The model under review builds one solid part; all positions refer to its coordinate system, in mm. A direction names the side the tool comes from. Round coordinates to 2 decimals unless told otherwise and drop trailing zeros. Order: outer loops, then holes, each group sorted by start corner. A loop starts at its lowest first (then second) coordinate and runs counter-clockwise, first axis right, second up.
from build123d import *

# Parameters (mm, degrees)
SKETCH_1_W           = 27
SKETCH_1_H           = 16.5
EXTRUDE_1_DEPTH      = 4
SKETCH_2_R           = 1.1
CUT_EXTRUDE_1_DEPTH  = 4
SKETCH_3_R           = 4.8
EXTRUDE_2_DEPTH      = 10
EXTRUDE_3_DEPTH      = 13
FILLET_1_R           = 0.5
FILLET_2_R           = 1
EXTRUDE_4_REACH      = 29.807
EXTRUDE_4_END_RADIUS = 4.8
SKETCH_7_R           = 1.3
CUT_EXTRUDE_3_DEPTH  = 7
CHAMFER_1_SIZE       = 0.4
CHAMFER_1_SIZE2      = 0.692820323
FILLET_3_R           = 0.5
EXTRUDE_5_DEPTH      = 14
FILLET_4_R           = 0.5
CHAMFER_2_SIZE       = 1


with BuildPart() as part:
    # Sketch 1 → Extrude 1 (new body)
    with BuildSketch(Plane.XY):
        with Locations((3.5, 0)):
            Rectangle(SKETCH_1_W, SKETCH_1_H)
    extrude(amount=EXTRUDE_1_DEPTH)

    # Sketch 2 → Cut-Extrude 1 (cut)
    with BuildSketch(Plane.XY.offset(4)):
        with Locations((-8, 0)):
            Circle(SKETCH_2_R)
        Circle(SKETCH_2_R)
    extrude(amount=-CUT_EXTRUDE_1_DEPTH, mode=Mode.SUBTRACT)



with BuildPart() as body_2:
    # Sketch 3 → Extrude 2 (new body)
    with BuildSketch(Plane.XZ.offset(8.25)):
        with Locations(Location((9.5, 12, 0), (0, 0, 270))):
            Circle(SKETCH_3_R)
    extrude(amount=-EXTRUDE_2_DEPTH)


with BuildPart() as part_1:
    add(part.part)

    add(body_2.part)  # Extrude 3 merges body 2
    # Sketch 4 → Extrude 3 (add)
    with BuildSketch(Plane.XZ.offset(8.25)):
        with BuildLine():
            Line((6.5, 4), (12.5, 4))
            Line((12.5, 4), (12.38, 8.16))
            ThreePointArc((12.38, 8.16), (9.5, 7.2), (6.62, 8.16))
            Line((6.62, 8.16), (6.5, 4))
        make_face()
    extrude(amount=-EXTRUDE_3_DEPTH)

    # Fillet 1
    fillet_1_edges = [part_1.edges().sort_by_distance(p)[0] for p in [
        (6.62, 3.25, 8.16),
        (12.38, 3.25, 8.16),
    ]]
    fillet(fillet_1_edges, radius=FILLET_1_R)

    # Fillet 2
    # the kernel refuses this fillet: 1 mm, written as the material it adds along each edge
    with BuildSketch(Plane(origin=(7.094742907, 1.75, 7.277210748), x_dir=(0.45382209295910925, 0, 0.891092311683932), z_dir=(0.891092311683932, 0, -0.45382209295910925))) as fillet_2_piece_1_section:
        with BuildLine():
            CenterArc((0.5 + FILLET_2_R, -FILLET_2_R), FILLET_2_R, 90, 90)
            Line((0.5, -FILLET_2_R), (0.5, 0))
            Line((0.5, 0), (0.5 + FILLET_2_R, 0))
        make_face()
    fillet_2_piece_1 = revolve(axis=Axis((7.094742907, 1.75, 7.277210748), (0, -1, 0)), revolution_arc=359.64, mode=Mode.PRIVATE)
    fillet_2_piece_1 = split(fillet_2_piece_1, bisect_by=Plane(origin=(6.594950803, 1.75, 7.291627828), z_dir=(0.9995842091710025, 0, -0.02883415987993323)), keep=Keep.TOP, mode=Mode.PRIVATE)
    add(fillet_2_piece_1)
    with BuildSketch(Plane(origin=(7.094742907, 1.75, 7.277210748), x_dir=(0.45382209295910925, 0, 0.891092311683932), z_dir=(0.891092311683932, 0, -0.45382209295910925))) as fillet_2_piece_2_section:
        with BuildLine():
            CenterArc((0.5 + FILLET_2_R, -FILLET_2_R), FILLET_2_R, 90, 90)
            Line((0.5, -FILLET_2_R), (0.5, 0))
            Line((0.5, 0), (0.5 + FILLET_2_R, 0))
        make_face()
    fillet_2_piece_2 = revolve(axis=Axis((7.094742907, 1.75, 7.277210748), (0, -1, 0)), revolution_arc=359.64, mode=Mode.PRIVATE)
    fillet_2_piece_2 = fillet_2_piece_2 & Plane(origin=(9.5, 1.75, 12), x_dir=(0.6, 0, -0.8000000000000002), z_dir=(0, -1, 0)) * Cylinder(4.8, 6, mode=Mode.PRIVATE)
    add(fillet_2_piece_2)
    with BuildSketch(Plane(origin=(11.905257093, 1.75, 7.277210748), x_dir=(-0.45941199618044226, 0, 0.8882232927397824), z_dir=(0.8882232927397824, 0, 0.45941199618044226))) as fillet_2_piece_3_section:
        with BuildLine():
            CenterArc((0.5 + FILLET_2_R, -FILLET_2_R), FILLET_2_R, 90, 90)
            Line((0.5 + FILLET_2_R, 0), (0.5, 0))
            Line((0.5, 0), (0.5, -FILLET_2_R))
        make_face()
    fillet_2_piece_3 = revolve(axis=Axis((11.905257093, 1.75, 7.277210748), (0, -1, 0)), revolution_arc=359.64, mode=Mode.PRIVATE)
    fillet_2_piece_3 = split(fillet_2_piece_3, bisect_by=Plane(origin=(12.405049197, 1.75, 7.291627828), z_dir=(-0.9995842091710025, 0, -0.02883415987993387)), keep=Keep.TOP, mode=Mode.PRIVATE)
    add(fillet_2_piece_3)
    with BuildSketch(Plane(origin=(11.905257093, 1.75, 7.277210748), x_dir=(-0.45941199618044226, 0, 0.8882232927397824), z_dir=(0.8882232927397824, 0, 0.45941199618044226))) as fillet_2_piece_4_section:
        with BuildLine():
            CenterArc((0.5 + FILLET_2_R, -FILLET_2_R), FILLET_2_R, 90, 90)
            Line((0.5 + FILLET_2_R, 0), (0.5, 0))
            Line((0.5, 0), (0.5, -FILLET_2_R))
        make_face()
    fillet_2_piece_4 = revolve(axis=Axis((11.905257093, 1.75, 7.277210748), (0, -1, 0)), revolution_arc=359.64, mode=Mode.PRIVATE)
    fillet_2_piece_4 = fillet_2_piece_4 & Plane(origin=(9.5, 1.75, 12), x_dir=(0.6, 0, -0.8000000000000002), z_dir=(0, -1, 0)) * Cylinder(4.8, 7, mode=Mode.PRIVATE)
    add(fillet_2_piece_4)
    with BuildSketch(Plane(origin=(9.5, 1.75, 12), x_dir=(-0.4538220929591119, 0, -0.8910923116839305), z_dir=(-0.8910923116839305, 0, 0.4538220929591119))) as fillet_2_piece_5:
        with BuildLine():
            CenterArc((4.8 - FILLET_2_R, -FILLET_2_R), FILLET_2_R, 0, 90)
            Line((4.8, -FILLET_2_R), (4.8, 0))
            Line((4.8, 0), (4.8 - FILLET_2_R, 0))
        make_face()
    revolve(axis=Axis((9.5, 1.75, 12), (0, -1, 0)), revolution_arc=53.978342396)

    # Extrude 4: up to this cylinder (the profile starts outside it)
    extrude_4_end = Plane(origin=(9.5, -4.045075, 12), z_dir=(0, -1, 0)) * Cylinder(EXTRUDE_4_END_RADIUS, 70.214, mode=Mode.PRIVATE)
    # Sketch 5 → Extrude 4 (add, up to the surface)
    with BuildSketch(Plane.XY.offset(20.4), mode=Mode.PRIVATE) as extrude_4_sk1:
        with BuildLine():
            Line((6.5, -8.25), (6.5, -2.25))
            ThreePointArc((6.5, -2.25), (9.5, 0.75), (12.5, -2.25))
            Line((12.5, -2.25), (12.5, -8.25))
            Line((12.5, -8.25), (6.5, -8.25))
        make_face()
    extrude_4_tool1 = extrude(extrude_4_sk1.sketch, amount=-EXTRUDE_4_REACH, mode=Mode.PRIVATE) - extrude_4_end
    add(extrude_4_tool1.solids().sort_by_distance((9.5, -4.045075, 20.4))[0])

    # Sketch 7 → Cut-Extrude 3 (cut)
    with BuildSketch(Plane.XY.offset(20.4)):
        with Locations((9.5, -2.25)):
            Circle(SKETCH_7_R)
    extrude(amount=-CUT_EXTRUDE_3_DEPTH, mode=Mode.SUBTRACT)

    # Chamfer 1
    chamfer_1_edges = [part_1.edges().sort_by_distance(p)[0] for p in [
        (8.2, -2.25, 20.4),
    ]]
    chamfer_1_side = [part_1.faces().sort_by_distance(p)[0] for p in [
        (9.5, -4.257679358, 20.4),
    ]]
    chamfer(chamfer_1_edges, length=CHAMFER_1_SIZE, length2=CHAMFER_1_SIZE2, reference=chamfer_1_side[0])

    # Fillet 3
    fillet_3_edges = [part_1.edges().sort_by_distance(p)[0] for p in [
        (6.5, -1.75, 4),
        (12.5, -1.75, 4),
    ]]
    fillet(fillet_3_edges, radius=FILLET_3_R)

    # Sketch 8 → Extrude 5 (add)
    with BuildSketch(Plane(origin=(17, 0, 0), x_dir=(0, 0, -1), z_dir=(1, 0, 0))):
        with BuildLine():
            Line((6.5, 1.75), (17.350889359, 1.75))
            ThreePointArc((17.350889359, 1.75), (18.144565149, 1.050392929), (17.550087952, 0.17519685))
            ThreePointArc((17.550087952, 0.17519685), (8.361036446, -3.17500409), (0, -8.25))
            Line((0, -8.25), (0, 8.25))
            Line((0, 8.25), (6.5, 1.75))
        make_face()
    extrude(amount=-EXTRUDE_5_DEPTH)

    # Fillet 4
    # the kernel refuses this fillet: 0.5 mm, written as the material it adds along each edge
    with BuildSketch(Plane(origin=(3, -8.25, 0), x_dir=(-1, 0, 0), z_dir=(0, 1, 0))) as fillet_4_piece_1_section:
        with BuildLine():
            CenterArc((FILLET_4_R, -FILLET_4_R), FILLET_4_R, 90, 90)
            Line((0, -FILLET_4_R), (0, 0))
            Line((0, 0), (FILLET_4_R, 0))
        make_face()
    fillet_4_piece_1 = extrude(amount=16.5, mode=Mode.PRIVATE)
    fillet_4_piece_1 = fillet_4_piece_1 - Plane(origin=(3, -48.25, -30), x_dir=(0, 0.9685039370078732, 0.24899824095814338), z_dir=(1, 0, 0)) * Cylinder(50, 35, mode=Mode.PRIVATE)
    fillet_4_piece_1 = split(fillet_4_piece_1, bisect_by=Plane(origin=(3, 0, -8.25), z_dir=(0, -0.7071067811865462, 0.7071067811865488)), keep=Keep.TOP, mode=Mode.PRIVATE)
    add(fillet_4_piece_1)

    # Chamfer 2
    chamfer_2_edges = [part_1.edges().sort_by_distance(p)[0] for p in [
        (-10, 8.25, 2),
        (17, 8.25, 2),
        (17, -8.25, 2),
        (-10, -8.25, 2),
    ]]
    chamfer(chamfer_2_edges, length=CHAMFER_2_SIZE)


solid = part_1.part
(1) To check wall thickness, follow L1, parallel to Y at x = 9.5, z = 17.25; L2, parallel to Y at x = -8, z = 1.85; L3, parallel to X at y = 1.5, z = -1.5. State the ranges of each line that lie inside material, in increasing order.
(2) Clearance check with flat-ended pins moving along their axes: P1, Ø3, axis at x = -5, y = 2, coming from the -Z side; P2, Ø5, axis at x = 1.5, y = -0.5, coming from the +Z side; P3, Ø4, axis at y = 4.5, z = 6.5, coming from the +X side; P4, Ø1.3, axis at x = 0, y = 0, coming from the +Z side. State where each tip first meets the part, or that it passes through.
(3) The part is to be moulded in two halves that separate along Z. For faces 1 (the flat face through (-4, 0, 0)), 2 (the cylindrical face through (5.6, -3.3, 9.2)), 3 (the flat face through (12.5, -5, 18)), 4 (the flat face through (10, -5, 20.4)), say which applies: pulls with the +Z half, pulls with the -Z half, needs draft (parallel to the pull), parting line crosses it, or undercut.
(4) We need section D-D (x = 9.5). Give the boundary of the cut face in (y, z).
(5) Tool access review of faces 5 (the flat face through (10, 1.75, -12)), 6 (the flat face through (6.5, -5, 18)), 7 (the cylindrical face through (9.5, 3.7, 7.2)): name each direction out of +Z, -Z, +X, -X, +Y, -Y from which nothing blocks a thin tool from reaching the whole face with its end or side.
(6) We need section B-B (x = 15.25). Give the boundary of the cut face in (y, z), and give its area (3 significant figures).
(7) We need section C-C (z = 12). Give the boundary of the cut face in (x, y), and give its area (3 significant figures).
(8) We need section A-A (x = 0). Give the boundary of the cut face in (y, z), and give its area (3 significant figures).
Verdict:
1. L1: y = -8.25 to -3.55, -0.95 to 0.75
1. L2: y = -8.25 to -1.1, 1.1 to 8.25
1. L3: x = 3 to 17
2. P1: stops at z = 0
2. P2: stops at z = 4
2. P3: stops at x = 12.49
2. P4: passes through
3. face 1: pulls with the -Z half
3. face 2: undercut
3. face 3: needs draft
3. face 4: pulls with the +Z half
4. outline: (-8.25, 0) arc R50 cw to (0.18, -17.55) arc R0.8 ccw to (1.75, -17.35) - (1.75, -6.5) - (8.25, 0) - (8.25, 4) - (4.75, 4) - (4.75, 7.2) - (2.75, 7.2) arc R1 cw to (1.75, 8.2) - (1.75, 16.8) - (0.75, 16.8) - (0.75, 20.4) - (-0.55, 20.4) - (-0.95, 19.71) - (-0.95, 13.4) - (-3.55, 13.4) - (-3.55, 19.71) - (-3.95, 20.4) - (-8.25, 20.4) - close
5. face 5: -Z, +X, -X, +Y
5. face 6: +Z, -X, +Y, -Y
5. face 7: +Z, +Y
6. outline: (-8.25, 0) arc R50 cw to (0.18, -17.55) arc R0.8 ccw to (1.75, -17.35) - (1.75, -6.5) - (8.25, 0) - (8.25, 4) - (-8.25, 4) - close
6. area: 177 mm2
7. outline: (4.7, -8.25) - (14.3, -8.25) - (14.3, 1.75) - (4.7, 1.75) - close
7. area: 96.0 mm2
8. outline: (-8.25, 0) - (-1.1, 0) - (-1.1, 4) - (-8.25, 4) - close; (1.1, 0) - (8.25, 0) - (8.25, 4) - (1.1, 4) - close
8. area: 57.2 mm2
